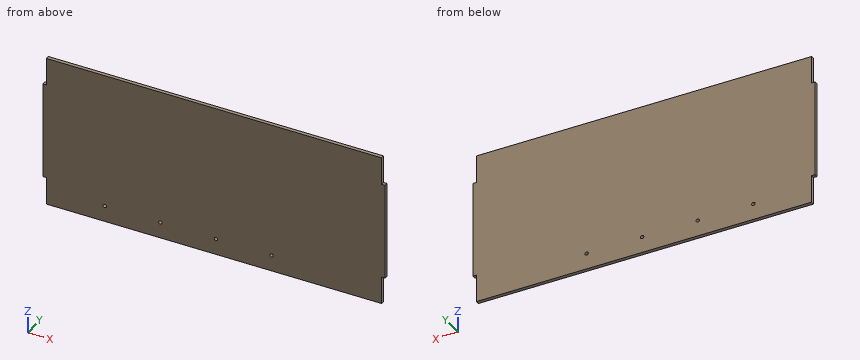
from build123d import *

# Parameters (mm, degrees)
BOSS_EXTRUDE1_DEPTH = 3.175
SKETCH3_R           = 1.5494
CUT_EXTRUDE1_DEPTH  = 170.119050616


with BuildPart() as part:
    # Sketch1 → Boss-Extrude1 (new body)
    with BuildSketch(Plane(origin=(0, 0, 0), x_dir=(1, 0, 0), z_dir=(0, 1, 0))):
        Polygon((-150.8125, 44.45), (-153.9875, 44.45), (-153.9875, -44.45), (-150.8125, -44.45), (-150.8125, -69.85), (150.8125, -69.85), (150.8125, -44.45), (153.9875, -44.45), (153.9875, 44.45), (150.8125, 44.45), (150.8125, 69.85), (-150.8125, 69.85), align=None)
    extrude(amount=BOSS_EXTRUDE1_DEPTH)

    # Sketch3 → Cut-Extrude1 (cut, through all)
    with BuildSketch(Plane(origin=(0, 3.175, 0), x_dir=(1, 0, 0), z_dir=(0, 1, 0))):
        with Locations(Location((-98.37039, 55.087774, 0), (0, 0, 270))):
            Circle(SKETCH3_R)
        with Locations(Location((-48.33239, 55.087774, 0), (0, 0, 270))):
            Circle(SKETCH3_R)
        with Locations(Location((1.70561, 55.087774, 0), (0, 0, 270))):
            Circle(SKETCH3_R)
        with Locations(Location((51.74361, 55.087774, 0), (0, 0, 270))):
            Circle(SKETCH3_R)
    extrude(amount=-CUT_EXTRUDE1_DEPTH, mode=Mode.SUBTRACT)


solid = part.part
The listing builds one solid part. Answer for the finished solid, in the listing's coordinates (mm). Coordinates: 2 decimals unless noted, no trailing zeros. Write each loop counter-clockwise with the first axis right and the second up, starting at its lowest first coordinate (ties: lowest second). Pieces come first, ordered by that corner, then holes. Notation, with made-up numbers: M 51.5,80 L 89.5,80 A15 cw 89.5,108 Z; hole C 54.25,14.5 d10. An arc over 180 degrees is marked long. Put each result on its own line as item: value. Start each with the question number.
1. Consider line 1 (X direction, y = 2.3, z = -60); line 2 (Z direction, x = -99, y = 1.9). Determine where each line is inside the solid, lowest interval first. Write a range as from..to.
2. A cutting plane is placed at A-A on z = -61. Write down the section's boundary in (x, y) (1 decimal), then the cut area to 3 significant figures.
3. Flat-ended cylindrical pins translate along their axes: P1, Ø1, axis at x = -152, y = 2.5, coming from the -Z side; P2, Ø1.6, axis at x = 152.5, y = 1, coming from the +Z side; P3, Ø1, axis at y = 2, z = -51.5, coming from the +X side; P4, Ø1.9, axis at x = 1.71, z = -55.09, coming from the -Y side. Find the tip coordinate at first contact, or state that the pin passes through.
Resolved:
1. line 1: x = -150.81..150.81
1. line 2: z = -69.85..-56.5, -53.67..69.85
2. outline: M -150.8,0 L 150.8,0 L 150.8,3.2 L -150.8,3.2 Z
2. area: 958 mm2
3. P1: stops at z = -44.45
3. P2: stops at z = 44.45
3. P3: stops at x = 150.81
3. P4: passes through
